Could you check a few things on this model? Use its own coordinates, in mm. Coordinates: 2 decimals unless noted, no trailing zeros. Write each loop counter-clockwise with the first axis right and the second up, starting at its lowest first coordinate (ties: lowest second). Pieces come first, ordered by that corner, then holes. Notation, with made-up numbers: M -25.75,67.25 L 26.25,67.25 A27 ccw 26.25,106.25 Z; hole C 83.25,57.25 d10. An arc over 180 degrees is marked long. Write item = value, one per line.
```python
from build123d import *

# Parameters (mm, degrees)
CROQUIS2_W                     = 179
CROQUIS2_H                     = 320
SALIENTE_EXTRUIR1_DEPTH        = 3
TALADRO_DE_MARGEN_PARA_M3_51_D = 3.9
CORTAR_EXTRUIR1_DEPTH          = 184.355528959
TALADRO_DE_MARGEN_PARA_M3_52_D = 3.9


with BuildPart() as part:
    # Croquis2 → Saliente-Extruir1 (new body)
    with BuildSketch(Plane.XY):
        Rectangle(CROQUIS2_W, CROQUIS2_H)
    extrude(amount=SALIENTE_EXTRUIR1_DEPTH)

    # Taladro de margen para M3.51 (through all)
    with Locations(Plane.XY.offset(3)):
        with Locations((0, 149), (-68.69, 49.42), (66.31, 49.42), (-68.69, -50.58), (0, -149), (66.31, -50.58)):
            Hole(TALADRO_DE_MARGEN_PARA_M3_51_D / 2)

    # robot arm bores → Cortar-Extruir1 (cut, through all)
    with BuildSketch(Plane.XY.offset(3)):
        with BuildLine():
            Line((-15, 45), (15, 45))
            ThreePointArc((15, 45), (20, 40), (15, 35))
            Line((15, 35), (-15, 35))
            ThreePointArc((-15, 35), (-20, 40), (-15, 45))
        make_face()
    extrude(amount=-CORTAR_EXTRUIR1_DEPTH, mode=Mode.SUBTRACT)

    # Taladro de margen para M3.52 (through all)
    with Locations(Plane.XY.offset(3)):
        with Locations((-24.154111306, 64.317986379), (25.673602741, 65.84242489), (24.14916423, 115.670138938), (-25.623407417, 111.66583138)):
            Hole(TALADRO_DE_MARGEN_PARA_M3_52_D / 2)


solid = part.part
```
Item 1: If I drill on line 1 along Y through (x, z) = (0, 2.1); line 2 along Y through (x, z) = (68, 1.55); line 3 along X through (y, z) = (149, 1.3), over which ranges is the centre line in solid material (lowest first)?
Numbers:
line_1 = -160 to -150.95, -147.05 to 35, 45 to 147.05, 150.95 to 160
line_2 = -160 to -51.55, -49.61 to 48.45, 50.39 to 160
line_3 = -89.5 to -1.95, 1.95 to 89.5
Item 2: Imagine slicing it at A-A (y = 40). Write out the boundary of the cut face in (x, z), and give its area (3 significant figures).
Numbers:
outline = M -89.5,0 L -20,0 L -20,3 L -89.5,3 Z; M 20,0 L 89.5,0 L 89.5,3 L 20,3 Z
area = 417 mm²
Item 3: I'm going to push a flat-ended pin straight in: P1, Ø10, axis at x = 2.5, y = -108.5, coming from the -Z side. Where does the tip first touch, or does it pass through?
Numbers:
P1 = 0
